Check sheet for the modelled part. Datum: model origin and axes. Units: mm. Give positions to 0.01 mm unless a question says otherwise; leave off trailing zeros. Write each loop counter-clockwise with the first axis right and the second up, starting at its lowest first coordinate (ties: lowest second). Pieces come first, ordered by that corner, then holes. Notation, with made-up numbers: (63.5, -39.5) -> (100.5, -39.5) arc R18 cw to (100.5, -24.5) -> close; hole circle Ø6 at (-2.75, 38). An arc over 180 degrees is marked (long way). Use a Markdown table: item, result. Add a question column.
1. Cross-section at B-B (z = 0). Enter the section's corners in (x, y), then the cut area to 3 significant figures.
2. Cross-section at A-A (y = 2.1). Enter the section's corners in (x, z).
3. Cross-section at C-C (x = 110). Enter the section's corners in (y, z), then the cut area to 3 significant figures.
4. Scan lines: probe 1 along Z at (x, y) = (0, 1.45); probe 2 along X at (y, z) = (1.35, 0); probe 3 along Z at (x, y) = (32, 1.85). Record each from-to range of solid material in increasing order. Write a range as [from, to].
5. Cross-section at D-D (z = 11). Enter the section's corners in (x, y).
from build123d import *

# Parameters (mm, degrees)
BOSS_EXTRUDE1_DEPTH = 3
CUT_EXTRUDE1_REACH  = 5
SKETCH2_R           = 2.159


with BuildPart() as part:
    # Sketch1 → Boss-Extrude1 (new body)
    with BuildSketch(Plane(origin=(0, 0, 0), x_dir=(1, 0, 0), z_dir=(0, 1, 0))):
        with BuildLine():
            Line((0, 5), (80, 5))
            ThreePointArc((80, 5), (100.801257358, -1.298113962), (114.615384615, -18.076923077))
            ThreePointArc((114.615384615, -18.076923077), (111.923076923, -24.615384615), (105.384615385, -21.923076923))
            ThreePointArc((105.384615385, -21.923076923), (95.254255396, -9.618616906), (80, -5))
            Line((80, -5), (0, -5))
            ThreePointArc((0, -5), (-5, 0), (0, 5))
        make_face()
    extrude(amount=BOSS_EXTRUDE1_DEPTH)

    # Sketch2 → Cut-Extrude1 (cut, up to next)
    with BuildSketch(Plane(origin=(0, 3, 0), x_dir=(1, 0, 0), z_dir=(0, 1, 0)), mode=Mode.PRIVATE) as cut_extrude1_sk1:
        Circle(SKETCH2_R)
    cut_extrude1_tool1 = extrude(cut_extrude1_sk1.sketch, amount=-CUT_EXTRUDE1_REACH, mode=Mode.PRIVATE) & part.part
    add(cut_extrude1_tool1.solids().sort_by_distance((0, 3, 0))[0], mode=Mode.SUBTRACT)


solid = part.part
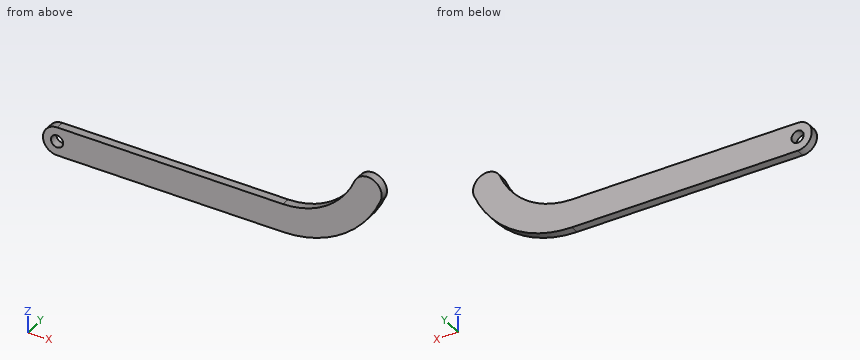
Worked answers:
| question | item | result |
|---|---|---|
| 1 | outline | (-5, 0) -> (-2.16, 0) -> (-2.16, 3) -> (-5, 3) -> close; (2.16, 0) -> (98.71, 0) -> (98.71, 3) -> (2.16, 3) -> close |
| 1 | area | 298 mm² |
| 2 | outline | (0, -5) -> (80, -5) arc R37.5 ccw to (114.62, 18.08) arc R5 ccw to (105.38, 21.92) arc R27.5 cw to (80, 5) -> (0, 5) arc R5 ccw to start; hole circle Ø4.32 at (0, 0) |
| 3 | outline | (0, 10) -> (3, 10) -> (3, 25) -> (0, 25) -> close |
| 3 | area | 45.0 mm² |
| 4 | probe 1 | z = [-5, -2.16], [2.16, 5] |
| 4 | probe 2 | x = [-5, -2.16], [2.16, 98.71] |
| 4 | probe 3 | z = [-5, 5] |
| 5 | outline | (97.15, 0) -> (110.72, 0) -> (110.72, 3) -> (97.15, 3) -> close |
